```python
from build123d import *

# Parameters (mm, degrees)
SKETCH2_W                = 198
SKETCH2_H                = 78
BOSS_EXTRUDE1_DEPTH      = 50
BOSS_EXTRUDE1_DEPTH_BACK = 15
SHELL1_T                 = -2
BOSS_EXTRUDE2_REACH      = 198
SKETCH3_W                = 2.5
SKETCH3_H                = 2
CUT_EXTRUDE1_REACH       = 4
CROQUIS1_W               = 35.265
CROQUIS1_H               = 26
SALIENTE_EXTRUIR1_DEPTH  = 38.9
CORTAR_EXTRUIR1_DEPTH    = 2
CORTAR_EXTRUIR2_DEPTH    = 30
CROQUIS5_W               = 26
CROQUIS5_H               = 15
CORTAR_EXTRUIR3_DEPTH    = 35.265
CROQUIS6_W               = 12
CROQUIS6_H               = 3
SALIENTE_EXTRUIR2_DEPTH  = 3
CROQUIS7_W               = 26
CROQUIS7_H               = 15
CORTAR_EXTRUIR4_DEPTH    = 35.265
CROQUIS8_W               = 12
CROQUIS8_H               = 3
SALIENTE_EXTRUIR4_DEPTH  = 3
CROQUIS10_W              = 12.009872988
CROQUIS10_H              = 3
SALIENTE_EXTRUIR5_DEPTH  = 3
CROQUIS11_W              = 12.098159715
CROQUIS11_H              = 3
SALIENTE_EXTRUIR6_DEPTH  = 3
CROQUIS12_W              = 11.962837464
CROQUIS12_H              = 3.064497362
SALIENTE_EXTRUIR7_DEPTH  = 3


with BuildPart() as part:
    # Sketch2 → Boss-Extrude1 (new body, two sides)
    with BuildSketch(Plane(origin=(0, 0, 0), x_dir=(1, 0, 0), z_dir=(0, 1, 0))) as boss_extrude1_sk:
        Rectangle(SKETCH2_W, SKETCH2_H)
    extrude(amount=BOSS_EXTRUDE1_DEPTH)
    extrude(boss_extrude1_sk.sketch, amount=-BOSS_EXTRUDE1_DEPTH_BACK)

    # Shell1
    shell1_openings = [part.faces().sort_by_distance(p)[0] for p in [
        (0, 50, 0),
    ]]
    offset(amount=SHELL1_T, openings=shell1_openings, kind=Kind.INTERSECTION)

    # Sketch3 → Boss-Extrude2 (add, up to next)
    with BuildSketch(Plane(origin=(-97, 0, 0), x_dir=(0, 0, -1), z_dir=(1, 0, 0)), mode=Mode.PRIVATE) as boss_extrude2_sk1:
        with Locations((-35.75, 49)):
            Rectangle(SKETCH3_W, SKETCH3_H)
    boss_extrude2_tool1 = extrude(boss_extrude2_sk1.sketch, amount=BOSS_EXTRUDE2_REACH, mode=Mode.PRIVATE) - part.part
    add(boss_extrude2_tool1.solids().sort_by_distance((-97, 49, 35.75))[0])
    # Sketch3 → Boss-Extrude2 (add, up to next)
    with BuildSketch(Plane(origin=(-97, 0, 0), x_dir=(0, 0, -1), z_dir=(1, 0, 0)), mode=Mode.PRIVATE) as boss_extrude2_sk2:
        with Locations((35.75, 49)):
            Rectangle(SKETCH3_W, SKETCH3_H)
    boss_extrude2_tool2 = extrude(boss_extrude2_sk2.sketch, amount=BOSS_EXTRUDE2_REACH, mode=Mode.PRIVATE) - part.part
    add(boss_extrude2_tool2.solids().sort_by_distance((-97, 49, -35.75))[0])

    # Sketch4 → Cut-Extrude1 (cut, up to next)
    with BuildSketch(Plane.ZY.offset(-97), mode=Mode.PRIVATE) as cut_extrude1_sk1:
        Polygon((-37, 48), (-37, 45), (-31.5, 45), (-31.5, 50), (-34.5, 50), (-34.5, 48), align=None)
    cut_extrude1_tool1 = extrude(cut_extrude1_sk1.sketch, amount=-CUT_EXTRUDE1_REACH, mode=Mode.PRIVATE) & part.part
    add(cut_extrude1_tool1.solids().sort_by_distance((97, 47.166667, -33.916667))[0], mode=Mode.SUBTRACT)
    # Sketch4 → Cut-Extrude1 (cut, up to next)
    with BuildSketch(Plane.ZY.offset(-97), mode=Mode.PRIVATE) as cut_extrude1_sk2:
        Polygon((34.5, 48), (37, 48), (37, 45), (31.5, 45), (31.5, 50), (34.5, 50), align=None)
    cut_extrude1_tool2 = extrude(cut_extrude1_sk2.sketch, amount=-CUT_EXTRUDE1_REACH, mode=Mode.PRIVATE) & part.part
    add(cut_extrude1_tool2.solids().sort_by_distance((97, 47.166667, 33.916667))[0], mode=Mode.SUBTRACT)

    # Croquis1 → Saliente-Extruir1 (add)
    with BuildSketch(Plane(origin=(0, -13, 0), x_dir=(1, 0, 0), z_dir=(0, 1, 0))):
        with Locations((79.3675, -16.5)):
            Rectangle(CROQUIS1_W, CROQUIS1_H)
    saliente_extruir1 = extrude(amount=SALIENTE_EXTRUIR1_DEPTH)

    # Simetría1: Saliente-Extruir1 across plane
    add(saliente_extruir1.mirror(Plane(origin=(0, 0, 0), x_dir=(0, 0, 1), z_dir=(1, 0, 0))))

    # Croquis2 → Cortar-Extruir1 (cut)
    with BuildSketch(Plane(origin=(0, 25.9, 0), x_dir=(1, 0, 0), z_dir=(0, 1, 0))):
        with BuildLine():
            Line((82.41, -12.375), (82.41, -20.625))
            ThreePointArc((82.41, -20.625), (79.235, -23.8), (76.06, -20.625))
            Line((76.06, -20.625), (76.06, -12.375))
            ThreePointArc((76.06, -12.375), (79.235, -9.2), (82.41, -12.375))
        make_face()
    cortar_extruir1 = extrude(amount=-CORTAR_EXTRUIR1_DEPTH, mode=Mode.SUBTRACT)

    # Simetría2: Cortar-Extruir1 across plane
    add(cortar_extruir1.mirror(Plane(origin=(0, 0, 0), x_dir=(0, 0, 1), z_dir=(1, 0, 0))), mode=Mode.SUBTRACT)

    # Croquis3 → Cortar-Extruir2 (cut)
    with BuildSketch(Plane(origin=(0, 23.9, 0), x_dir=(1, 0, 0), z_dir=(0, 1, 0))):
        with BuildLine():
            Line((80.835, -13.2), (80.835, -19.8))
            ThreePointArc((80.835, -19.8), (79.235, -21.4), (77.635, -19.8))
            Line((77.635, -19.8), (77.635, -13.2))
            ThreePointArc((77.635, -13.2), (79.235, -11.6), (80.835, -13.2))
        make_face()
    cortar_extruir2 = extrude(amount=-CORTAR_EXTRUIR2_DEPTH, mode=Mode.SUBTRACT)

    # Simetría3: Cortar-Extruir2 across plane
    add(cortar_extruir2.mirror(Plane(origin=(0, 0, 0), x_dir=(0, 0, 1), z_dir=(1, 0, 0))), mode=Mode.SUBTRACT)

    # Croquis5 → Cortar-Extruir3 (cut)
    with BuildSketch(Plane.ZY.offset(-61.735)):
        with Locations((16.5, -5.5)):
            Rectangle(CROQUIS5_W, CROQUIS5_H)
    extrude(amount=-CORTAR_EXTRUIR3_DEPTH, mode=Mode.SUBTRACT)

    # Croquis6 → Saliente-Extruir2 (add)
    with BuildSketch(Plane.ZY.offset(-61.735)):
        with Locations((16.5, 3.5)):
            Rectangle(CROQUIS6_W, CROQUIS6_H)
    saliente_extruir2 = extrude(amount=SALIENTE_EXTRUIR2_DEPTH)

    # Croquis7 → Cortar-Extruir4 (cut)
    with BuildSketch(Plane(origin=(-61.735, 0, 0), x_dir=(0, 0, -1), z_dir=(1, 0, 0))):
        with Locations((-16.5, -5.5)):
            Rectangle(CROQUIS7_W, CROQUIS7_H)
    extrude(amount=-CORTAR_EXTRUIR4_DEPTH, mode=Mode.SUBTRACT)

    # Simetría7: Saliente-Extruir2 across plane
    add(saliente_extruir2.mirror(Plane(origin=(0, 0, 0), x_dir=(0, 0, 1), z_dir=(1, 0, 0))))

    # Croquis8 → Saliente-Extruir4 (add)
    with BuildSketch(Plane.XY.offset(-37)):
        with Locations((91, 3.5)):
            Rectangle(CROQUIS8_W, CROQUIS8_H)
    extrude(amount=SALIENTE_EXTRUIR4_DEPTH)

    # Croquis10 → Saliente-Extruir5 (add)
    with BuildSketch(Plane.ZY.offset(-97)):
        with Locations((-30.995063506, 3.5)):
            Rectangle(CROQUIS10_W, CROQUIS10_H)
    extrude(amount=SALIENTE_EXTRUIR5_DEPTH)

    # Croquis11 → Saliente-Extruir6 (add)
    with BuildSketch(Plane.XY.offset(-37)):
        with Locations((-90.950920142, 3.5)):
            Rectangle(CROQUIS11_W, CROQUIS11_H)
    extrude(amount=SALIENTE_EXTRUIR6_DEPTH)

    # Croquis12 → Saliente-Extruir7 (add)
    with BuildSketch(Plane(origin=(-97, 0, 0), x_dir=(0, 0, -1), z_dir=(1, 0, 0))):
        with Locations((31.018581268, 3.467751319)):
            Rectangle(CROQUIS12_W, CROQUIS12_H)
    extrude(amount=SALIENTE_EXTRUIR7_DEPTH)


solid = part.part
```
Design review of the part built by this model. Coordinates are the model's own, in mm. A direction names the side the tool comes from. Coordinates: 2 decimals unless noted, no trailing zeros. Order: outer loops, then holes, each group sorted by start corner. A loop starts at its lowest first (then second) coordinate and runs counter-clockwise, first axis right, second up.
1) Take a section at B-B, the plane z = 27. Give the boundary of the cut face in (x, y) (3 decimals), and give its area (3 significant figures).
2) Mouldability with a two-part tool opening along Z and no side actions: class faces 4 (the flat face through (-1, 18, 39)), 5 (the flat face through (-1, -15, -1)), 6 (the flat face through (-61.735, 14, 17)) as +Z half, -Z half, draft (parallel to the pull), parting line (faces both ways), or undercut.
3) Take a section at C-C, the plane x = 24. Give the boundary of the cut face in (y, z).
4) Wall thickness on line 1 along X through (y, z) = (5.5, -23); line 2 along Z through (x, y) = (-2.5, 2); line 3 along X through (y, z) = (8, 7) (3 decimals): over which ranges is each line inside the solid? List them lowest first.
5) Take a section at A-A, the plane y = 43. Give the boundary of the cut face in (x, z).
6) For faces 1 (the flat face through (99, 18, 1)), 2 (the flat face through (-77, 23.9, 16)), 3 (the flat face through (-1, -13, -1)), list the 3-axis set-ups (+Z, -Z, +X, -X, +Y, -Y) from which the entire face can be reached by the end or side of a thin tool; tool diameter is ignored.
7) Take a section at D-D, the plane y = 14. Give the boundary of the cut face in (x, z) (3 decimals), and give its area (3 significant figures).
Returned:
1. outline: (-99, -15) - (99, -15) - (99, 50) - (97, 50) - (97, 25.9) - (61.735, 25.9) - (61.735, 2) - (97, 2) - (97, -13) - (-97, -13) - (-97, 2) - (-61.735, 2) - (-61.735, 25.9) - (-97, 25.9) - (-97, 50) - (-99, 50) - close
1. area: 2,330 mm2
2. face 4: +Z half
2. face 5: draft
2. face 6: undercut
3. outline: (-15, -39) - (50, -39) - (50, -34.5) - (48, -34.5) - (48, -37) - (-13, -37) - (-13, 37) - (48, 37) - (48, 34.5) - (50, 34.5) - (50, 39) - (-15, 39) - close
4. line 1: x = -99 to -97, 97 to 99
4. line 2: z = -39 to -37, 37 to 39
4. line 3: x = -99 to -61.735, 61.735 to 99
5. outline: (-99, -39) - (99, -39) - (99, 39) - (-99, 39) - close; hole (-97, -37) - (97, -37) - (97, 37) - (-97, 37) - close
6. face 1: +Z, -Z, +X, +Y, -Y
6. face 2: +Y
6. face 3: none
7. outline: (-99, -39) - (99, -39) - (99, 39) - (-99, 39) - close; hole (-97, -37) - (97, -37) - (97, 3.5) - (61.735, 3.5) - (61.735, 29.5) - (97, 29.5) - (97, 37) - (-97, 37) - (-97, 29.5) - (-61.735, 29.5) - (-61.735, 3.5) - (-97, 3.5) - close; hole (-80.835, 13.2) arc R1.6 ccw to (-77.635, 13.2) - (-77.635, 19.8) arc R1.6 ccw to (-80.835, 19.8) - close; hole (77.635, 13.2) arc R1.6 ccw to (80.835, 13.2) - (80.835, 19.8) arc R1.6 ccw to (77.635, 19.8) - close
7. area: 2,860 mm2
